Input: part model. Units: mm. Frame: model coordinates. A direction names the side the tool comes from. Give positions to 0.01 mm unless a question says otherwise; leave off trailing zeros. Loops run counter-clockwise (first coordinate to the right, second up) from the corner with the lowest first, then second, coordinate; pieces in that order, holes last. Notation, with made-up numbers: M 50,23.5 L 68,23.5 A13 ccw 68,32.5 Z; hole C -37.5,-35 d10. An arc over 180 degrees is marked long. Use a Markdown table: item, result. Add a question column.
from build123d import *

# Parameters (mm, degrees)
CYLINDER002_R           = 1.8
CYLINDER002_DEPTH       = 10
ARRAY003_X_COUNT        = 2
ARRAY003_X_PITCH        = 75
ARRAY003_Y_COUNT        = 2
ARRAY003_Y_PITCH        = 31
BOX008_W                = 80.4
BOX008_H                = 36.4
BOX008_DEPTH            = 4.7
BOX_W                   = 71.2
BOX_H                   = 25
BOX_DEPTH               = 3.8
BODY001_PLACEMENT_ANGLE = 115


with BuildPart() as hole_clone:
    # Cylinder002 → Cylinder002 (new body)
    with BuildSketch(Plane(origin=(3.7, 3.7, 0), x_dir=(1, 0, 0), z_dir=(0, 0, 1))):
        Circle(CYLINDER002_R)
    extrude(amount=CYLINDER002_DEPTH)

    # Array003 X: hole clone ×2


with BuildPart() as hole_clone_1:
    add(hole_clone.part)
    with Locations(*[(i * ARRAY003_X_PITCH, 0, 0) for i in range(1, ARRAY003_X_COUNT)]):
        add(hole_clone.part)

    # Array003 Y: hole clone ×2


with BuildPart() as hole_clone_2:
    add(hole_clone_1.part)
    with Locations(*[(0, i * ARRAY003_Y_PITCH, 0) for i in range(1, ARRAY003_Y_COUNT)]):
        add(hole_clone_1.part)


with BuildPart() as hole_clone_3:
    # Body placement: moved
    add(hole_clone_2.part.moved(Location((-1, -1, 0))))


with BuildPart() as under_display:
    # Box008 → Box008 (new body)
    with BuildSketch(Plane.XY):
        with Locations((40.2, 18.2)):
            Rectangle(BOX008_W, BOX008_H)
    extrude(amount=BOX008_DEPTH)


with BuildPart() as f_16x2_lcd_clone:
    # Box → Box (new body)
    with BuildSketch(Plane(origin=(4.4, 5.2, 4.7), x_dir=(1, 0, 0), z_dir=(0, 0, 1))):
        with Locations((35.6, 12.5)):
            Rectangle(BOX_W, BOX_H)
    extrude(amount=BOX_DEPTH)

    # Fusion004: union under display
    add(under_display.part)

    # Cut: cut hole clone
    add(hole_clone_3.part, mode=Mode.SUBTRACT)


with BuildPart() as f_16x2_lcd_clone_1:
    # Body001 placement: moved
    add(f_16x2_lcd_clone.part.moved(Location((1, 21.460623, -9.855736))).rotate(Axis((1, 21.460623, -9.855736), (-1, 0, 0)), BODY001_PLACEMENT_ANGLE))


solid = f_16x2_lcd_clone_1.part
1) Section query C-C, the plane y = 9. State how many separate pieces and enclosed holes the cut face has, and give its area (3 significant figures).
2) Section query A-A, the plane x = 25. Return the cut outline in (y, z), and give its area (3 significant figures).
3) Section query B-B, the plane y = 18.5. Return the cut outline in (x, z).
4) Contact query for flat-ended pins moving along their axis: P1, Ø4, axis at y = 22, z = -27, coming from the +X side; P2, Ø12, axis at x = 55, z = -19.5, coming from the -Y side; P3, Ø8, axis at x = 68.5, y = 12, coming from the -Z side. Output: stop coordinate, or through.
5) Reachability of faces 4 (the flat face through (76.6, 20, -29)), 5 (the flat face through (40.502, 25.221, -17.347)), 6 (the flat face through (5.4, 20, -29)) from +Z, -Z, +X, -X, +Y, -Y: full face, straight path, thin tool, end or side. Return the list, or none.
6) Ray query, line 1 (X direction, y = 23, z = -12); line 2 (X direction, y = 22.5, z = -12.5); line 3 (X direction, y = 22.5, z = -23.5). Return the intervals inside material, ascending. Write a range as [from, to].
7) Pull-direction query (Z, two-part tool) for faces 1 (the flat face through (40.637, 23.561, -10.835)), 2 (the flat face through (40.637, 8.177, -43.825)), 3 (the cylindrical face through (2.373, 8.804, -42.48)); classes: pulls with the +Z half, pulls with the -Z half, needs draft (parallel to the pull), parting line crosses it, or undercut.
Entries:
| question | item | result |
|---|---|---|
| 1 | separate pieces | 1 |
| 1 | enclosed holes | 2 |
| 1 | area | 591 mm² |
| 2 | outline | M 6.08,-42.85 L 10.34,-44.83 L 12.96,-39.21 L 16.4,-40.82 L 26.97,-18.16 L 23.52,-16.55 L 25.72,-11.84 L 21.46,-9.86 Z |
| 2 | area | 266 mm² |
| 3 | outline | M 1,-27.33 L 5.4,-27.33 L 5.4,-36.32 L 76.6,-36.32 L 76.6,-27.33 L 81.4,-27.33 L 81.4,-16.2 L 1,-16.2 Z |
| 4 | P1 | stops at x = 76.6 |
| 4 | P2 | stops at y = 14.17 |
| 4 | P3 | stops at z = -44.83 |
| 5 | face 4 | -Z, +X, +Y |
| 5 | face 5 | +X, -X, +Y |
| 5 | face 6 | -Z, -X, +Y |
| 6 | line 1 | x = [1, 2.58], [4.82, 77.58], [79.82, 81.4] |
| 6 | line 2 | x = [1, 2.06], [5.34, 77.06], [80.34, 81.4] |
| 6 | line 3 | x = [5.4, 76.6] |
| 7 | face 1 | pulls with the +Z half |
| 7 | face 2 | pulls with the -Z half |
| 7 | face 3 | undercut |
